The listing builds one solid part. Answer for the finished solid, in the listing's coordinates (mm). Face numbers are marked on the shaded views. A direction names the side the tool comes from. Round coordinates to 2 decimals unless told otherwise and drop trailing zeros. Loops run counter-clockwise (first coordinate to the right, second up) from the corner with the lowest first, then second, coordinate; pieces in that order, holes last. Notation, with made-up numbers: (-27, -4) -> (13, -4) arc R30 cw to (13, 34) -> close; hole circle Ø11 at (-5.75, 38). An arc over 180 degrees is marked (long way). Use a Markdown table: item, result. Add a question column.
Q1. Which of the six approach directions +Z, -Z, +X, -X, +Y, -Y give full straight-line access (tool end or side, diameter ignored) to the marked faces 1, 2 and 3?
Q2. Consider line 1 (Y direction, x = 14.88, z = 6.2); line 2 (Y direction, x = -13, z = 3.75); line 3 (X direction, y = 15, z = 1). Determine where each line is inside the solid, lowest interval first.
Q3. Section B-B on y = 15.5 is taken. Give the number of separate pieces and of enclosed holes in the cut face, then the cut area to 3 significant figures.
Q4. Given pin 1 Ø6 at (x, y) = (6.5, -4) entering from +Z; pin 2 Ø2 at (x, z) = (0.5, 2.5) entering from -Y; pin 3 Ø5.5 at (x, y) = (0, 15.5) entering from -Z, each flat-ended and moving along its own axis, determine where each tip first touches the part or whether it passes through.
Q5. For a pull along Y with two mould halves and no side action, classify the marked faces 4, 5 and 6 as released by +Y, released by -Y, zero draft, split by the parting line, or undercut.
Q6. Section C-C on x = 7 is taken. Give the vertices of the cut face in (y, z), then the cut area to 3 significant figures.
Q7. Section A-A on x = 0 is taken. Give the vertices of the cut face in (y, z), then the cut area to 3 significant figures.
from build123d import *

# Parameters (mm, degrees)
CROQUIS1_W              = 40
CROQUIS1_H              = 45
SALIENTE_EXTRUIR1_DEPTH = 8
CROQUIS2_W              = 31
CROQUIS2_H              = 1.3
CORTAR_EXTRUIR1_DEPTH   = 6.6
CROQUIS3_R              = 15
CORTAR_EXTRUIR2_DEPTH   = 10
CHAFL_N1_SIZE           = 2
CROQUIS4_W              = 27
CROQUIS4_H              = 28
CORTAR_EXTRUIR3_DEPTH   = 6.6
CROQUIS6_R              = 2.75
CORTAR_EXTRUIR4_DEPTH   = 16.6
CROQUIS7_R              = 1.65
CORTAR_EXTRUIR5_DEPTH   = 16.6
CROQUIS8_R              = 4
CORTAR_EXTRUIR6_DEPTH   = 4
CROQUIS9_W              = 18
CROQUIS9_H              = 6.6
CORTAR_EXTRUIR7_DEPTH   = 4
REDONDEO1_R             = 1
REDONDEO2_R             = 2
REDONDEO3_R             = 1
REDONDEO4_R             = 3
REDONDEO5_R             = 0.5
REDONDEO6_R             = 0.5


with BuildPart() as part:
    # Croquis1 → Saliente-Extruir1 (new body)
    with BuildSketch(Plane.XY):
        Rectangle(CROQUIS1_W, CROQUIS1_H)
    extrude(amount=SALIENTE_EXTRUIR1_DEPTH)

    # Croquis2 → Cortar-Extruir1 (cut)
    with BuildSketch(Plane.XY.offset(8)):
        with Locations((0, -21.15)):
            Rectangle(CROQUIS2_W, CROQUIS2_H)
    extrude(amount=-CORTAR_EXTRUIR1_DEPTH, mode=Mode.SUBTRACT)

    # Croquis3 → Cortar-Extruir2 (cut)
    with BuildSketch(Plane.XY.offset(8)):
        with Locations((-30, -6.5)):
            Circle(CROQUIS3_R)
        with Locations((30, -6.5)):
            Circle(CROQUIS3_R)
    extrude(amount=-CORTAR_EXTRUIR2_DEPTH, mode=Mode.SUBTRACT)

    # Chaflán1
    chafl_n1_edges = [part.edges().sort_by_distance(p)[0] for p in [
        (-15, -6.5, 0),
        (15, -6.5, 0),
    ]]
    chamfer(chafl_n1_edges, length=CHAFL_N1_SIZE)

    # Croquis4 → Cortar-Extruir3 (cut)
    with BuildSketch(Plane.XY.offset(8)):
        with Locations((0, -6.5)):
            Rectangle(CROQUIS4_W, CROQUIS4_H)
    extrude(amount=-CORTAR_EXTRUIR3_DEPTH, mode=Mode.SUBTRACT)

    # Croquis6 → Cortar-Extruir4 (cut)
    with BuildSketch(Plane(origin=(0, 22.5, 0), x_dir=(1, 0, 0), z_dir=(0, 1, 0))):
        with Locations((7, -8)):
            Circle(CROQUIS6_R)
        with Locations((-7, -8)):
            Circle(CROQUIS6_R)
    extrude(amount=-CORTAR_EXTRUIR4_DEPTH, mode=Mode.SUBTRACT)

    # Croquis7 → Cortar-Extruir5 (cut)
    with BuildSketch(Plane.XY.offset(8)):
        with Locations((0, 15.5)):
            Circle(CROQUIS7_R)
        with Locations((14.88, 15.5)):
            Circle(CROQUIS7_R)
        with Locations((-14.875, 15.5)):
            Circle(CROQUIS7_R)
    extrude(amount=-CORTAR_EXTRUIR5_DEPTH, mode=Mode.SUBTRACT)

    # Croquis8 → Cortar-Extruir6 (cut)
    with BuildSketch(Plane(origin=(0, 0, 0), x_dir=(-1, 0, 0), z_dir=(0, 0, -1))):
        with Locations((14.875, 15.5)):
            Circle(CROQUIS8_R)
        with Locations((0, 15.5)):
            Circle(CROQUIS8_R)
        with Locations((-14.88, 15.5)):
            Circle(CROQUIS8_R)
    extrude(amount=-CORTAR_EXTRUIR6_DEPTH, mode=Mode.SUBTRACT)

    # Croquis9 → Cortar-Extruir7 (cut)
    with BuildSketch(Plane(origin=(0, -22.5, 0), x_dir=(-1, 0, 0), z_dir=(0, -1, 0))):
        with Locations((0, -4.7)):
            Rectangle(CROQUIS9_W, CROQUIS9_H)
    extrude(amount=-CORTAR_EXTRUIR7_DEPTH, mode=Mode.SUBTRACT)

    # Redondeo1
    redondeo1_edges = [part.edges().sort_by_distance(p)[0] for p in [
        (7, 22.5, 5.25),
        (-7, 22.5, 5.25),
    ]]
    fillet(redondeo1_edges, radius=REDONDEO1_R)

    # Redondeo2
    redondeo2_edges = [part.edges().sort_by_distance(p)[0] for p in [
        (-20, 22.5, 4),
        (20, 22.5, 4),
    ]]
    fillet(redondeo2_edges, radius=REDONDEO2_R)

    # Redondeo3
    redondeo3_edges = [part.edges().sort_by_distance(p)[0] for p in [
        (20, -22.5, 4),
        (-20, -22.5, 4),
    ]]
    fillet(redondeo3_edges, radius=REDONDEO3_R)

    # Redondeo4
    redondeo4_edges = [part.edges().sort_by_distance(p)[0] for p in [
        (7, 7.5, 5.25),
        (-7, 7.5, 5.25),
    ]]
    fillet(redondeo4_edges, radius=REDONDEO4_R)

    # Redondeo5
    redondeo5_edges = [part.edges().sort_by_distance(p)[0] for p in [
        (13.5, -20.5, 4.7),
        (-13.5, -20.5, 4.7),
    ]]
    fillet(redondeo5_edges, radius=REDONDEO5_R)

    # Redondeo6
    redondeo6_edges = [part.edges().sort_by_distance(p)[0] for p in [
        (-13.5, 7.5, 4.7),
        (13.5, 7.5, 4.7),
    ]]
    fillet(redondeo6_edges, radius=REDONDEO6_R)


solid = part.part
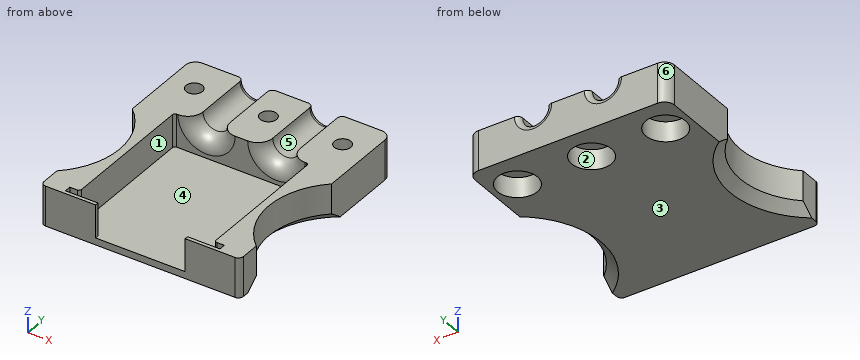
Checked values:
| question | item | result |
|---|---|---|
| 1 | face 1 | +Z |
| 1 | face 2 | -Z |
| 1 | face 3 | -Z, +X, -X, +Y, -Y |
| 2 | line 1 | y = -22.5 to -21.8, -20.5 to 13.85, 17.15 to 22.5 |
| 2 | line 2 | y = -22.5 to -21.8, 7.5 to 11.97, 19.03 to 22.5 |
| 2 | line 3 | x = -20 to -18.84, -10.91 to -3.97, 3.97 to 10.91, 18.85 to 20 |
| 3 | separate pieces | 4 |
| 3 | enclosed holes | 0 |
| 3 | area | 161 mm2 |
| 4 | pin 1 | stops at z = 1.4 |
| 4 | pin 2 | stops at y = 7.5 |
| 4 | pin 3 | stops at z = 4 |
| 5 | face 4 | undercut |
| 5 | face 5 | zero draft |
| 5 | face 6 | released by +Y |
| 6 | outline | (-22.5, 0) -> (22.5, 0) -> (22.5, 4.25) arc R1 ccw to (21.5, 5.25) -> (10.5, 5.25) arc R3 ccw to (7.5, 2.25) -> (7.5, 1.4) -> (-22.5, 1.4) -> close |
| 6 | area | 119 mm2 |
| 7 | outline | (-22.5, 0) -> (11.5, 0) -> (11.5, 4) -> (13.85, 4) -> (13.85, 8) -> (7.5, 8) -> (7.5, 1.4) -> (-22.5, 1.4) -> close; (17.15, 4) -> (19.5, 4) -> (19.5, 0) -> (22.5, 0) -> (22.5, 8) -> (17.15, 8) -> close |
| 7 | area | 117 mm2 |
